Build history of the part. All positions in model axes, mm. A direction names the side the tool comes from. Give positions to 0.01 mm unless a question says otherwise; leave off trailing zeros. Loops run counter-clockwise (first coordinate to the right, second up) from the corner with the lowest first, then second, coordinate; pieces in that order, holes last. Notation, with made-up numbers: M 70.25,35.25 L 93.25,35.25 A25 cw 93.25,60.25 Z; hole C 2,7 d10. An arc over 180 degrees is marked long. Put each result on its own line as item: value.
Autodesk Inventor part; units mm, degrees
ref_plane "YZ Plane" through (0, 0, 0) normal (1, 0, 0) x (0, 1, 0)
ref_plane "XZ Plane" through (0, 0, 0) normal (0, 1, 0) x (-1, 0, 0)
ref_plane "XY Plane" through (0, 0, 0) normal (0, 0, 1) x (1, 0, 0)
sketch "Sketch9" plane through (0, 0, 0) normal (0, 1, 0) x (-1, 0, 0)
  line L0 (0, 0) -> (-20, 0)
  line L1 (-20, 0) -> (-20, -47)
  line L2 (-20, -47) -> (0, -47)
  line L3 (0, -47) -> (0, 0)
  dimension "d20" = 20
  dimension "d21" = 47
extrude "Extrusion6" add sketch "Sketch9" along normal blind 2
sketch "Sketch10" plane through (0, 0, 0) normal (0, 0, 1) x (1, 0, 0)
  line L0 (0, 0) -> (20, 0)
  line L1 (0, 0) -> (20, 0)
  line L2 (20, 0) -> (20, 30)
  line L3 (20, 30) -> (0, 30)
  line L4 (0, 30) -> (0, 0)
  dimension "d24" = 30
  dimension "d40" = 20
extrude "Extrusion7" add sketch "Sketch10" along normal blind 2
sketch "Sketch11" plane through (20, 0, -47) normal (0, 0, -1) x (-1, 0, 0)
  line L0 (0, 2) -> (0, 30)
  line L1 (0, 0) -> (20, 0)
  line L2 (0, 30) -> (20, 30)
  line L3 (20, 30) -> (20, 0)
  line L4 (20, 0) -> (0, 0)
  line L5 (0, 0) -> (0, 30)
  dimension "d39" = 30
extrude "Extrusion8" add sketch "Sketch11" along normal blind 2
sketch "Sketch12" plane through (20, 0, -49) normal (0, 0, -1) x (-1, 0, 0)
  circle A0 centre (10, 24.36) radius 0.75
  line L0 (20, 30) -> (0, 30)
  line L1 (0, 30) -> (0, 0)
  point P0 (20, 0)
  dimension "d29" = 1.5
  dimension "d30" = 5.64
  dimension "d31" = 10
extrude "Extrusion9" cut sketch "Sketch12" against normal blind 2
sketch "Sketch13" plane through (20, 0, -49) normal (0, 0, -1) x (-1, 0, 0)
  circle A0 centre (10, 16.86) radius 0.75
  line L0 (0, 30) -> (0, 0)
  circle A1 centre (10, 24.36) radius 0.75
  point P0 (20, 0)
  dimension "d34" = 1.5
  dimension "d35" = 10
  dimension "d36" = 7.5
extrude "Extrusion10" cut sketch "Sketch13" against normal blind 2 contours A0
sketch "Sketch14" plane through (0, 0, 0) normal (0, -1, 0) x (1, 0, 0)
  circle A0 centre (10, -23.5) radius 0.75
  line L0 (0, 2) -> (0, -49)
  line L1 (20, -47) -> (0, -47)
  circle A1 centre (10, -30.6) radius 0.75
  circle A2 centre (10, -16.4) radius 0.75
  point P0 (0, 0)
  dimension "d41" = 1.5
  dimension "d42" = 10
  dimension "d43" = 23.5
  dimension "d44" = 1.5
  dimension "d45" = 7.1
  dimension "d46" = 1.5
  dimension "d47" = 7.1
extrude "Extrusion11" cut sketch "Sketch14" against normal blind 10
sketch "Sketch15" plane through (0, 0, 2) normal (0, 0, 1) x (1, 0, 0)
  circle A0 centre (10, 24.36) radius 0.75
  circle A1 centre (10, 24.36) radius 0.75
  circle A2 centre (10, 16.86) radius 0.75
  circle A3 centre (10, 16.86) radius 0.75
  point P0 (0, 0)
extrude "Extrusion12" cut sketch "Sketch15" against normal blind 2
properties part number "Servo Holder Upper Part"
Q1. Mould opens along Z. For faces 1 (the cylindrical face through (9.45, 24.87, 1.01)), 2 (the cylindrical face through (9.837, 0.986, -31.332)), 3 (the flat face through (10, 15, 2)) say: pulls with the +Z half, pulls with the -Z half, needs draft (parallel to the pull), parting line crosses it, or undercut.
Here are the results:
face 1: needs draft
face 2: undercut
face 3: pulls with the +Z half
Q2. Slice it at A-A (y = 21). List the corners of the cut face in (x, z).
Here are the results:
outline: M 0,-49 L 20,-49 L 20,-47 L 0,-47 Z; M 0,0 L 20,0 L 20,2 L 0,2 Z
Q3. Slice it at C-C (y = 24.36). List the corners of the cut face in (x, z).
Here are the results:
outline: M 0,-49 L 9.25,-49 L 9.25,-47 L 0,-47 Z; M 0,0 L 9.25,0 L 9.25,2 L 0,2 Z; M 10.75,-49 L 20,-49 L 20,-47 L 10.75,-47 Z; M 10.75,0 L 20,0 L 20,2 L 10.75,2 Z
Q4. Drop a flat-ended pin along its axis: pin 1 Ø2 at (x, z) = (10, -30.6) entering from +Y. Give the stop position or say it passes through.
Here are the results:
pin 1: y = 2
Q5. Probe line 1 (Y direction, x = 10, z = -48.1); line 2 (Z direction, x = 10, y = 0.85); line 3 (Z direction, x = 17.25, y = 15). List the from-to ranges inside material, lowest first. Write a range as from..to.
Here are the results:
line 1: 0..16.11, 17.61..23.61, 25.11..30
line 2: -49..-31.35, -29.85..-24.25, -22.75..-17.15, -15.65..2
line 3: -49..-47, 0..2
Q6. Slice it at D-D (x = 15.5). List the corners of the cut face in (y, z), and give its area (3 significant figures).
Here are the results:
outline: M 0,-49 L 30,-49 L 30,-47 L 2,-47 L 2,0 L 30,0 L 30,2 L 0,2 Z
area: 214 mm²
Q7. Slice it at B-B (z = -30.6). List the corners of the cut face in (x, y), and give its area (3 significant figures).
Here are the results:
outline: M 0,0 L 9.25,0 L 9.25,2 L 0,2 Z; M 10.75,0 L 20,0 L 20,2 L 10.75,2 Z
area: 37.0 mm²
Q8. Tool access for faces 4 (the flat face through (12, 0, -23)), 5 (the flat face through (12, 16, -47)): list every direction of +Z, -Z, +X, -X, +Y, -Y with a clear straight run to the whole face (end or side of a thin tool).
Here are the results:
face 4: +Z, -Z, +X, -X, -Y
face 5: +X, -X, +Y
